Geometry: final body of the model. Coordinates: model frame, mm. Face numbers are marked on the shaded views. A direction names the side the tool comes from. Coordinates: 2 decimals unless noted, no trailing zeros. Write each loop counter-clockwise with the first axis right and the second up, starting at its lowest first coordinate (ties: lowest second). Pieces come first, ordered by that corner, then holes.
from build123d import *

# Parameters (mm, degrees)
F0_R          = 10.5
F0_R_2        = 8.25
F1_DEPTH      = 22
F0_W          = 0.5
F0_H          = 3
F0_R_3        = 3
F2_DEPTH      = 25
F0_R_4        = 1
F3_DEPTH      = 27
F3_DEPTH_BACK = 2
F4_DEPTH      = 35
F4_DEPTH_BACK = 2.5
F5_DEPTH      = 5


with BuildPart() as f1:
    # F0 (on Front) → F1 (new body)
    with BuildSketch(Plane.XZ):
        Circle(F0_R)
        Circle(F0_R_2, mode=Mode.SUBTRACT)
    extrude(amount=F1_DEPTH)

    # F0 (on Front) → F2 (join)
    with BuildSketch(Plane.XZ):
        Circle(F0_R_2)
        with Locations((-7.75, 0)):
            Rectangle(F0_W, F0_H, mode=Mode.SUBTRACT)
        Circle(F0_R_3, mode=Mode.SUBTRACT)
        with Locations((7.75, 0)):
            Rectangle(F0_W, F0_H, mode=Mode.SUBTRACT)
        with Locations((-7.75, 0)):
            Rectangle(F0_W, F0_H)
        with Locations((7.75, 0)):
            Rectangle(F0_W, F0_H)
    extrude(amount=F2_DEPTH)

    # F0 (on Front) → F3 (join, two sides)
    with BuildSketch(Plane.XZ) as f3_sk:
        Circle(F0_R_3)
        Circle(F0_R_4, mode=Mode.SUBTRACT)
    extrude(amount=F3_DEPTH)
    extrude(f3_sk.sketch, amount=-F3_DEPTH_BACK)

    # F0 (on Front) → F4 (join, two sides)
    with BuildSketch(Plane.XZ) as f4_sk:
        Circle(F0_R_4)
    extrude(amount=F4_DEPTH)
    extrude(f4_sk.sketch, amount=-F4_DEPTH_BACK)

    # F0 (on Front) → F5 (join)
    with BuildSketch(Plane.XZ):
        with Locations((-7.75, 0)):
            Rectangle(F0_W, F0_H)
        with Locations((7.75, 0)):
            Rectangle(F0_W, F0_H)
    extrude(amount=-F5_DEPTH)


solid = f1.part
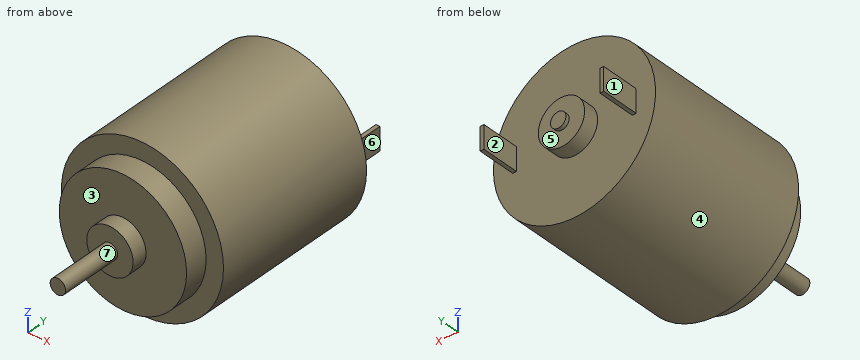
Item 1: Set-up query: the marked faces 4, 5, 6 and 7. Return all of +Z, -Z, +X, -X, +Y, -Y with unobstructed straight access to the full face (end or side cutting, diameter ignored); none if empty.
Derived:
face 4: +Y, -Y
face 5: +Y
face 6: +Z, -Z, +X, +Y
face 7: -Y
Item 2: Material intervals for probe 1 along Y at (x, z) = (-1, 3.25); probe 2 along Y at (x, z) = (-0.75, 1); probe 3 along X at (y, z) = (-13, 3.75), sorted ascending.
Derived:
probe 1: y = -25 to 0
probe 2: y = -27 to 2
probe 3: x = -9.81 to 9.81
Item 3: Section C-C, the plane y = -28.5. Output: boundary loops of the cut face in (x, z), plus the area to 3 significant figures.
Derived:
outline: circle Ø2 at (0, 0)
area: 3.14 mm2
Item 4: Pin query (flat end, axial travel): pin 1 (0.6 mm diameter, centred on x = 7.5, y = 2.5, fed in from -Z); pin 2 (6 mm diameter, centred on x = 1.5, z = 3.5, fed in from +Y); pin 3 (5 mm diameter, centred on x = -6.5, y = -22, fed in from -Z). Return the tip coordinate at first contact, or that it passes through.
Derived:
pin 1: stops at z = -1.5
pin 2: stops at y = 2.5
pin 3: stops at z = -9.71
Item 5: Pull-direction query (X, two-part tool) for the marked faces 1, 2 and 3; classes: released by +X, released by -X, zero draft, split by the parting line, or undercut.
Derived:
face 1: released by -X
face 2: undercut
face 3: zero draft
Item 6: Section A-A, the plane x = 0. Output: boundary loops of the cut face in (y, z).
Derived:
outline: (-35, -1) - (-27, -1) - (-27, -3) - (-25, -3) - (-25, -8.25) - (-22, -8.25) - (-22, -10.5) - (0, -10.5) - (0, -3) - (2, -3) - (2, -1) - (2.5, -1) - (2.5, 1) - (2, 1) - (2, 3) - (0, 3) - (0, 10.5) - (-22, 10.5) - (-22, 8.25) - (-25, 8.25) - (-25, 3) - (-27, 3) - (-27, 1) - (-35, 1) - close
Item 7: Section D-D, the plane x = 4.5. Output: boundary loops of the cut face in (y, z).
Derived:
outline: (-25, -6.91) - (-22, -6.91) - (-22, -9.49) - (0, -9.49) - (0, 9.49) - (-22, 9.49) - (-22, 6.91) - (-25, 6.91) - close
